Work out the finished part from the listing and answer in its coordinate system (mm). Face numbers are marked on the shaded views. A direction names the side the tool comes from. Give positions to 0.01 mm unless a question says otherwise; leave off trailing zeros. Write each loop counter-clockwise with the first axis right and the second up, starting at its lowest first coordinate (ties: lowest second). Pieces come first, ordered by that corner, then holes.
1) Straight lines are drawn through the part: probe 1 along X at (y, z) = (9.75, 0) (3 decimals); probe 2 along X at (y, z) = (20, 0) (3 decimals); probe 3 along X at (y, z) = (27.5, 0). For each, find the intervals that lie inside material, in ascending order.
2) A tool of negligible diameter and unlimited length cuts with its end or side. For the marked faces 5, 6 and 7, from which of +Z, -Z, +X, -X, +Y, -Y can it reach the whole face along a straight path? Write none if from no direction.
3) Find section A-A (z = 0). Count the separate pieces of the cut face and the enclosed holes in it, plus the area to 3 significant figures.
4) Find section B-B (x = 0). Determine the outline of the cut face in (y, z).
5) Determine the mould class of the marked faces 1, 2, 3 and 4 for opening direction Z: pulls with the +Z half, pulls with the -Z half, needs draft (parallel to the pull), parting line crosses it, or undercut.
6) Find section C-C (y = 46). Determine the outline of the cut face in (x, z).
7) Given pin 1 Ø23.5 at (x, z) = (75.5, 9) entering from +Y; pin 2 Ø2 at (x, y) = (-41, 34.5) entering from -Z; pin 3 Ø1 at (y, z) = (34.5, 26.5) entering from -X, each flat-ended and moving along its own axis, determine where each tip first touches the part or whether it passes through.
8) Find section D-D (x = -87.5). Determine the outline of the cut face in (y, z) (3 decimals), plus the area to 3 significant figures.
```python
from build123d import *

# Parameters (mm, degrees)
BOSS_EXTRUDE1_DEPTH   = 12
BOSS_EXTRUDE1_2_DEPTH = 12
BOSS_EXTRUDE2_DEPTH   = 9
SKETCH1_4_R           = 52.5
SKETCH1_4_R_2         = 40.5
BOSS_EXTRUDE3_DEPTH   = 63
SKETCH1_5_R           = 23.665
SKETCH1_5_R_2         = 11.665
BOSS_EXTRUDE4_DEPTH   = 25


with BuildPart() as part:
    # Sketch1 → Boss-Extrude1 (new body)
    with BuildSketch(Plane(origin=(0, 0, 0), x_dir=(1, 0, 0), z_dir=(0, 1, 0))):
        with BuildLine():
            Line((95.298631714, 22.343087709), (17.301, 49.56738241))
            ThreePointArc((17.301, 49.56738241), (42.805096075, 30.396936523), (52.5, 0))
            ThreePointArc((52.5, 0), (42.805096075, -30.396936523), (17.301, -49.56738241))
            Line((17.301, -49.56738241), (95.298631714, -22.343087709))
            ThreePointArc((95.298631714, -22.343087709), (63.835, 0), (95.298631714, 22.343087709))
        make_face()
        with BuildLine():
            ThreePointArc((73.102729075, -20.639666056), (74.665998298, -24.211578828), (72.196764974, -27.229070884))
            Line((72.196764974, -27.229070884), (51.320741116, -34.515638607))
            ThreePointArc((51.320741116, -34.515638607), (46.457803099, -33.130049608), (46.122102919, -28.084722223))
            ThreePointArc((46.122102919, -28.084722223), (53.990744033, 0.999779365), (45.050715916, 29.773024628))
            ThreePointArc((45.050715916, 29.773024628), (45.21504533, 34.020913269), (49.292435481, 35.22359844))
            Line((49.292435481, 35.22359844), (73.061565244, 26.927220983))
            ThreePointArc((73.061565244, 26.927220983), (75.234080861, 24.22863303), (73.769413903, 21.089054754))
            ThreePointArc((73.769413903, 21.089054754), (62.338211107, 0.40200089), (73.102729075, -20.639666056))
        make_face(mode=Mode.SUBTRACT)
    extrude(amount=BOSS_EXTRUDE1_DEPTH)



with BuildPart() as body_2:
    # Sketch1 → Boss-Extrude1 2 (new body)
    with BuildSketch(Plane(origin=(0, 0, 0), x_dir=(1, 0, 0), z_dir=(0, 1, 0))):
        with BuildLine():
            ThreePointArc((-17.301, -49.56738241), (-52.5, 0), (-17.301, 49.56738241))
            Line((-17.301, 49.56738241), (-95.298631714, 22.343087709))
            ThreePointArc((-95.298631714, 22.343087709), (-73.798218994, 19.29490664), (-63.835, 0))
            ThreePointArc((-63.835, 0), (-73.798218994, -19.29490664), (-95.298631714, -22.343087709))
            Line((-95.298631714, -22.343087709), (-17.301, -49.56738241))
        make_face()
        with BuildLine():
            Line((-73.061565244, 26.927220983), (-49.292435481, 35.22359844))
            ThreePointArc((-49.292435481, 35.22359844), (-45.21504533, 34.020913269), (-45.050715916, 29.773024628))
            ThreePointArc((-45.050715916, 29.773024628), (-53.990744033, 0.999779365), (-46.122102919, -28.084722223))
            ThreePointArc((-46.122102919, -28.084722223), (-46.457803099, -33.130049608), (-51.320741116, -34.515638607))
            Line((-51.320741116, -34.515638607), (-72.196764974, -27.229070884))
            ThreePointArc((-72.196764974, -27.229070884), (-74.665998298, -24.211578828), (-73.102729075, -20.639666056))
            ThreePointArc((-73.102729075, -20.639666056), (-62.338211107, 0.40200089), (-73.769413903, 21.089054754))
            ThreePointArc((-73.769413903, 21.089054754), (-75.234080861, 24.22863303), (-73.061565244, 26.927220983))
        make_face(mode=Mode.SUBTRACT)
    extrude(amount=BOSS_EXTRUDE1_2_DEPTH)


with BuildPart() as part_1:
    add(part.part)

    add(body_2.part)  # Boss-Extrude2 merges body 2
    # Sketch1_3 → Boss-Extrude2 (add)
    with BuildSketch(Plane(origin=(0, 0, 0), x_dir=(1, 0, 0), z_dir=(0, 1, 0))):
        with BuildLine():
            ThreePointArc((49.292435481, 35.22359844), (45.21504533, 34.020913269), (45.050715916, 29.773024628))
            ThreePointArc((45.050715916, 29.773024628), (53.990744033, 0.999779365), (46.122102919, -28.084722223))
            ThreePointArc((46.122102919, -28.084722223), (46.457803099, -33.130049608), (51.320741116, -34.515638607))
            Line((51.320741116, -34.515638607), (72.196764974, -27.229070884))
            ThreePointArc((72.196764974, -27.229070884), (74.665998298, -24.211578828), (73.102729075, -20.639666056))
            ThreePointArc((73.102729075, -20.639666056), (62.338211107, 0.40200089), (73.769413903, 21.089054754))
            ThreePointArc((73.769413903, 21.089054754), (75.234080861, 24.22863303), (73.061565244, 26.927220983))
            Line((73.061565244, 26.927220983), (49.292435481, 35.22359844))
        make_face()
        with BuildLine():
            Line((-72.196764974, -27.229070884), (-51.320741116, -34.515638607))
            ThreePointArc((-51.320741116, -34.515638607), (-46.457803099, -33.130049608), (-46.122102919, -28.084722223))
            ThreePointArc((-46.122102919, -28.084722223), (-53.990744033, 0.999779365), (-45.050715916, 29.773024628))
            ThreePointArc((-45.050715916, 29.773024628), (-45.21504533, 34.020913269), (-49.292435481, 35.22359844))
            Line((-49.292435481, 35.22359844), (-73.061565244, 26.927220983))
            ThreePointArc((-73.061565244, 26.927220983), (-75.234080861, 24.22863303), (-73.769413903, 21.089054754))
            ThreePointArc((-73.769413903, 21.089054754), (-62.338211107, 0.40200089), (-73.102729075, -20.639666056))
            ThreePointArc((-73.102729075, -20.639666056), (-74.665998298, -24.211578828), (-72.196764974, -27.229070884))
        make_face()
    extrude(amount=BOSS_EXTRUDE2_DEPTH)

    # Sketch1_4 → Boss-Extrude3 (add)
    with BuildSketch(Plane(origin=(0, 0, 0), x_dir=(1, 0, 0), z_dir=(0, 1, 0))):
        with Locations(Location((0, 0, 0), (0, 0, 109.241031138))):
            Circle(SKETCH1_4_R)
        with Locations(Location((0, 0, 0), (0, 0, 270))):
            Circle(SKETCH1_4_R_2, mode=Mode.SUBTRACT)
    extrude(amount=BOSS_EXTRUDE3_DEPTH)

    # Sketch1_5 → Boss-Extrude4 (add)
    # profile 1 of 2: a face of its own
    with BuildSketch(Plane(origin=(0, 0, 0), x_dir=(1, 0, 0), z_dir=(0, 1, 0))):
        with Locations(Location((-87.5, 0, 0), (0, 0, 109.241031138))):
            Circle(SKETCH1_5_R)
        with Locations(Location((-87.5, 0, 0), (0, 0, 270))):
            Circle(SKETCH1_5_R_2, mode=Mode.SUBTRACT)
    # profile 2 of 2: a face of its own
    with BuildSketch(Plane(origin=(0, 0, 0), x_dir=(1, 0, 0), z_dir=(0, 1, 0))):
        with Locations(Location((87.5, 0, 0), (0, 0, 70.758968862))):
            Circle(SKETCH1_5_R)
        with Locations(Location((87.5, 0, 0), (0, 0, 270))):
            Circle(SKETCH1_5_R_2, mode=Mode.SUBTRACT)
    extrude(amount=BOSS_EXTRUDE4_DEPTH)


solid = part_1.part
```
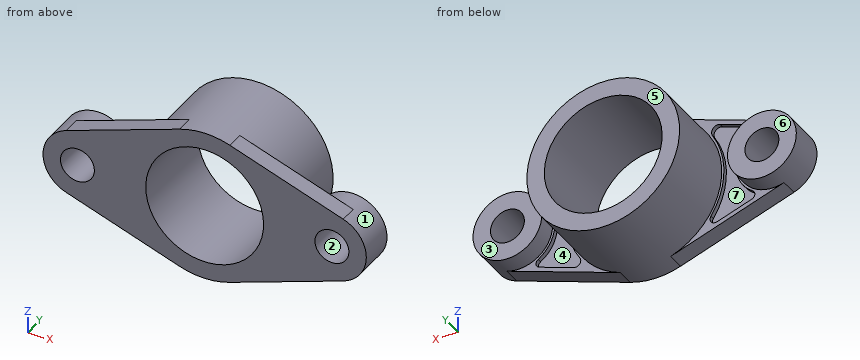
Results:
1. probe 1: x = -111.165 to -99.165, -75.835 to -62.335, -54 to -40.5, 40.5 to 54, 62.335 to 75.835, 99.165 to 111.165
1. probe 2: x = -111.165 to -99.165, -75.835 to -63.835, -52.5 to -40.5, 40.5 to 52.5, 63.835 to 75.835, 99.165 to 111.165
1. probe 3: x = -52.5 to -40.5, 40.5 to 52.5
2. face 5: +Z, -Z, +X, -X, +Y
2. face 6: +Z, -Z, -X, +Y
2. face 7: +Y
3. separate pieces: 4
3. enclosed holes: 0
3. area: 2,930 mm2
4. outline: (0, -52.5) - (63, -52.5) - (63, -40.5) - (0, -40.5) - close; (0, 40.5) - (63, 40.5) - (63, 52.5) - (0, 52.5) - close
5. face 1: parting line crosses it
5. face 2: undercut
5. face 3: needs draft
5. face 4: undercut
6. outline: circle Ø105 at (0, 0); hole circle Ø81 at (0, 0)
7. pin 1: stops at y = 25
7. pin 2: stops at z = -34
7. pin 3: stops at x = -45.61
8. outline: (0, -25.065) - (12, -25.065) - (12, -23.665) - (25, -23.665) - (25, -11.665) - (0, -11.665) - close; (0, 11.665) - (25, 11.665) - (25, 23.665) - (12, 23.665) - (12, 25.065) - (0, 25.065) - close
8. area: 634 mm2
